Autodesk Inventor part; units mm, degrees
ref_plane "YZ Plane" through (0, 0, 0) normal (1, 0, 0) x (0, 1, 0)
ref_plane "XZ Plane" through (0, 0, 0) normal (0, 1, 0) x (-1, 0, 0)
ref_plane "XY Plane" through (0, 0, 0) normal (0, 0, 1) x (1, 0, 0)
sketch "Sketch1" plane through (0, 0, 0) normal (0, 0, 1) x (1, 0, 0)
  circle A0 centre (0, 0) radius 9.525
  dimension "d0" = 19.05
extrude "Extrusion1" add sketch "Sketch1" along normal blind 1.5875
sketch "Sketch2" plane through (0, 0, 1.5875) normal (0, 0, 1) x (1, 0, 0)
  circle A0 centre (0, 0) radius 9.525
  circle A1 centre (0, 0) radius 3.9688
  dimension "d3" = 7.9375
extrude "Extrusion2" add sketch "Sketch2" along normal blind 7.9375 contours A1
hole "Hole1" at (0, 0, 9.525) direction (0, 0, -1) diameter 6.35 depth 25.4 tip angle 118
thread "Thread1"
fillet "Fillet1" radius 1.5875 1 edges at (0, 3.175, 0)
fillet "Fillet2" radius 0.254 2 edges at (-3.9688, 0, 9.525) (-9.525, 0, 0)
properties part number "Deck_Nut"
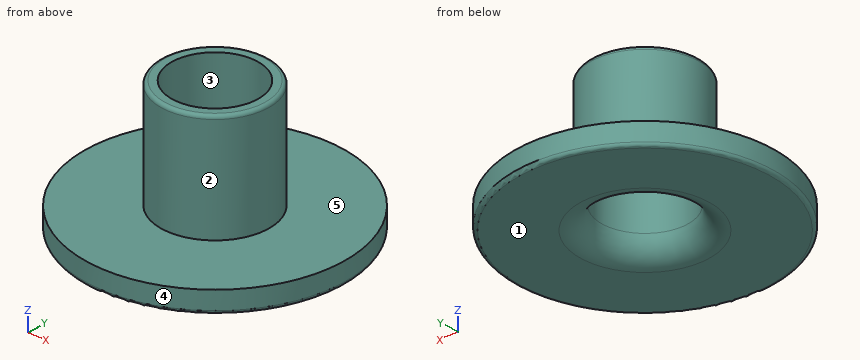
Source: CAD feature listing. Evaluate the final solid. Frame: model axes, mm. Face numbers are marked on the shaded views. A direction names the side the tool comes from. Give positions to 0.01 mm unless a question says otherwise; leave off trailing zeros. Order: outer loops, then holes, each group sorted by start corner. A loop starts at its lowest first (then second) coordinate and runs counter-clockwise, first axis right, second up. Notation, with made-up numbers: (84.25, 73) -> (105.25, 73) arc R16 cw to (105.25, 101) -> close; hole circle Ø1 at (51, 66). An arc over 180 degrees is marked (long way). Use a Markdown table: item, result.
Q1. Section C-C (z = 4). Return the cut outline in (x, y) (3 decimals), and give its area (3 significant figures).
A:
| item | result |
|---|---|
| outline | circle Ø7.938 at (0, 0); hole circle Ø6.35 at (0, 0) |
| area | 17.8 mm^2 |
Q2. Material intervals for line 1 (Y direction, x = 0, z = 4.5) (3 decimals); line 2 (Z direction, x = -4.5, y = -3); line 3 (X direction, y = -2.25, z = 3.25), sorted ascending. Write a range as [from, to].
A:
| item | result |
|---|---|
| line 1 | [-3.969, -3.175], [3.175, 3.969] |
| line 2 | [0, 1.59] |
| line 3 | [-3.27, -2.24], [2.24, 3.27] |
Q3. First-contact query: P1, Ø2, axis at x = -6, y = -4.5, coming from the +Z side; P2, Ø1.5, axis at x = 7, z = 2, coming from the -Y side; P3, Ø5, axis at x = -1.5, z = 6, coming from the +Y side; P4, Ø5.5, axis at x = 0, y = 0, coming from the +Z side. Flat tips, straight axial feed; report the tip coordinate or a pass-through.
A:
| item | result |
|---|---|
| P1 | z = 1.59 |
| P2 | y = -7.08 |
| P3 | y = 3.97 |
| P4 | through |
Q4. Pull-direction query (Y, two-part tool) for the marked faces 3, 4 and 5; classes: +Y half, -Y half, draft (parallel to the pull), parting line (faces both ways), or undercut.
A:
| item | result |
|---|---|
| face 3 | undercut |
| face 4 | parting line |
| face 5 | draft |
Q5. Access query for the marked faces 1 and 2. Directions: +Z, -Z, +X, -X, +Y, -Y. A direction counts if a zero-diameter tool reaches every point of the face in a straight line with its end or side. Return the directions, or none.
A:
| item | result |
|---|---|
| face 1 | -Z, +X, -X, +Y, -Y |
| face 2 | +Z |
